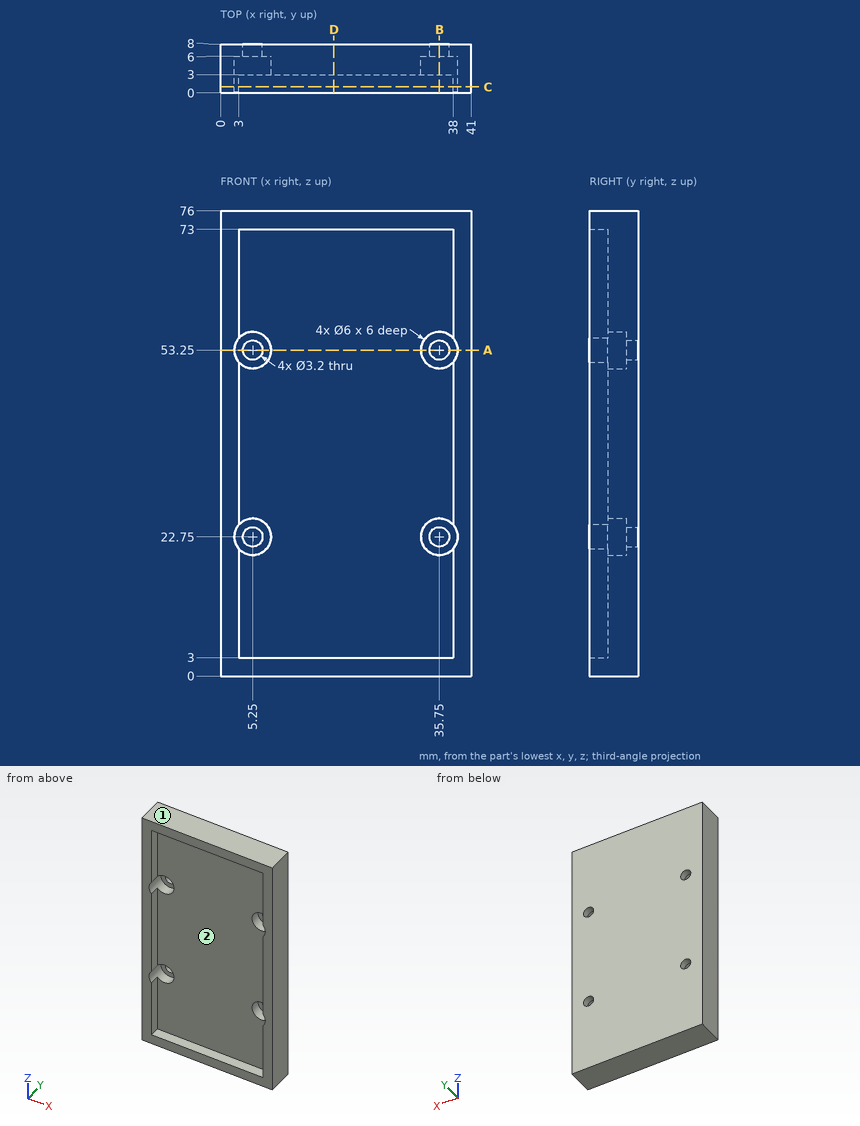
Design review of the part shown in the three views and the two pictorial views. Dimensions are in mm from the part's minimum x, y and z. Round coordinates to 2 decimals unless told otherwise and drop trailing zeros. Order: outer loops, then holes, each group sorted by start corner. A loop starts at its lowest first (then second) coordinate and runs counter-clockwise, first axis right, second up. Notation, with made-up numbers: (75, -19) - (122, -19) arc R27 ccw to (122, 17) - close; hole circle Ø6 at (-24.5, 48.25). An arc over 180 degrees is marked (long way). Answer in a Markdown table with one row per item.
(1) Take a section at C-C on y = 1. Write out the cut boundary in (x, z), plus the area to 3 significant figures.
Result set:
| item | result |
|---|---|
| outline | (0, 0) - (41, 0) - (41, 76) - (0, 76) - close; hole (3, 3) - (38, 3) - (38, 20.77) arc R3 ccw to (38, 24.73) - (38, 51.27) arc R3 ccw to (38, 55.23) - (38, 73) - (3, 73) - (3, 55.23) arc R3 ccw to (3, 51.27) - (3, 24.73) arc R3 ccw to (3, 20.77) - close |
| area | 658 mm2 |
(2) For line 1 (X direction, y = 6.55, z = 22.75); line 2 (Z direction, x = 35.75, y = 7.4); line 3 (Z direction, x = 33.5, y = 3.25), list the stretches that pass through material, from the lowest coordinate up. Write a range as from..to.
Result set:
| item | result |
|---|---|
| line 1 | x = 0..3.65, 6.85..34.15, 37.35..41 |
| line 2 | z = 0..21.15, 24.35..51.65, 54.85..76 |
| line 3 | z = 0..20.77, 24.73..51.27, 55.23..76 |
(3) Mouldability with a two-part tool opening along X and no side actions: class the marked faces 1 and 2 as released by +X, released by -X, zero draft, split by the parting line, or undercut.
Result set:
| item | result |
|---|---|
| face 1 | zero draft |
| face 2 | undercut |
(4) Take a section at D-D on x = 18.5. Write out the cut boundary in (y, z).
Result set:
| item | result |
|---|---|
| outline | (0, 0) - (8, 0) - (8, 76) - (0, 76) - (0, 73) - (3, 73) - (3, 3) - (0, 3) - close |
(5) Take a section at A-A on z = 53.25. Write out the cut boundary in (x, y), plus the area to 3 significant figures.
Result set:
| item | result |
|---|---|
| outline | (0, 0) - (2.25, 0) - (2.25, 6) - (3.65, 6) - (3.65, 8) - (0, 8) - close; (6.85, 6) - (8.25, 6) - (8.25, 3) - (32.75, 3) - (32.75, 6) - (34.15, 6) - (34.15, 8) - (6.85, 8) - close; (37.35, 6) - (38.75, 6) - (38.75, 0) - (41, 0) - (41, 8) - (37.35, 8) - close |
| area | 170 mm2 |
(6) Take a section at B-B on x = 35.75. Write out the cut boundary in (y, z).
Result set:
| item | result |
|---|---|
| outline | (0, 0) - (8, 0) - (8, 21.15) - (6, 21.15) - (6, 19.75) - (3, 19.75) - (3, 3) - (0, 3) - close; (0, 73) - (3, 73) - (3, 56.25) - (6, 56.25) - (6, 54.85) - (8, 54.85) - (8, 76) - (0, 76) - close; (3, 25.75) - (6, 25.75) - (6, 24.35) - (8, 24.35) - (8, 51.65) - (6, 51.65) - (6, 50.25) - (3, 50.25) - close |
(7) Clearance check with flat-ended pins moving along their axes: P1, Ø3.5, axis at x = 35.75, z = 53.25, coming from the -Y side; P2, Ø1.5, axis at y = 2, z = 15, coming from the -X side; P3, Ø4, axis at x = 8, z = 61.5, coming from the -Y side. State where each tip first meets the part, or that it passes through.
Result set:
| item | result |
|---|---|
| P1 | stops at y = 6 |
| P2 | stops at x = 0 |
| P3 | stops at y = 3 |
